```python
from build123d import *

# Parameters (mm, degrees)
SKETCH1_R           = 14.2875
BOSS_EXTRUDE1_DEPTH = 33.3375
SKETCH2_R           = 16.66875
BOSS_EXTRUDE2_DEPTH = 4.7625
FILLET1_R           = 3.175
SKETCH3_R           = 11.3109375
BOSS_EXTRUDE3_DEPTH = 4.7625
CUT_EXTRUDE1_START  = -4.7625
CUT_EXTRUDE1_DEPTH  = 4.7625


with BuildPart() as part:
    # Sketch1 → Boss-Extrude1 (new body)
    with BuildSketch(Plane.XY):
        Circle(SKETCH1_R)
    extrude(amount=BOSS_EXTRUDE1_DEPTH)

    # Sketch2 → Boss-Extrude2 (add)
    with BuildSketch(Plane(origin=(0, 0, 0), x_dir=(-1, 0, 0), z_dir=(0, 0, -1))):
        with Locations(Location((0, 0, 0), (0, 0, 180))):
            Circle(SKETCH2_R)
    extrude(amount=BOSS_EXTRUDE2_DEPTH)

    # Fillet1
    fillet1_edges = [part.edges().sort_by_distance(p)[0] for p in [
        (-16.66875, 0, -4.7625),
    ]]
    fillet(fillet1_edges, radius=FILLET1_R)

    # Sketch3 → Boss-Extrude3 (add)
    with BuildSketch(Plane(origin=(0, 0, -4.7625), x_dir=(-1, 0, 0), z_dir=(0, 0, -1))):
        with Locations(Location((0, 0, 0), (0, 0, 180))):
            Circle(SKETCH3_R)
    extrude(amount=BOSS_EXTRUDE3_DEPTH)

    # Sketch4 → Cut-Extrude1 (cut)
    with BuildSketch(Plane.XY.offset(33.3375).offset(CUT_EXTRUDE1_START)):
        with BuildLine():
            Line((-7.540625, 12.135552351), (-6.074392361, 9.775861616))
            ThreePointArc((-6.074392361, 9.775861616), (0, 11.509375), (6.074392361, 9.775861616))
            Line((6.074392361, 9.775861616), (7.540625, 12.135552351))
            ThreePointArc((7.540625, 12.135552351), (14.2875, 0), (7.540625, -12.135552351))
            Line((7.540625, -12.135552351), (6.074392361, -9.775861616))
            ThreePointArc((6.074392361, -9.775861616), (0, -11.509375), (-6.074392361, -9.775861616))
            Line((-6.074392361, -9.775861616), (-7.540625, -12.135552351))
            ThreePointArc((-7.540625, -12.135552351), (-14.2875, 0), (-7.540625, 12.135552351))
        make_face()
    extrude(amount=CUT_EXTRUDE1_DEPTH, mode=Mode.SUBTRACT)


solid = part.part
```
Can you work these out from the model? Positions are in its coordinate system, mm. A direction names the side the tool comes from. Round coordinates to 2 decimals unless told otherwise and drop trailing zeros. Loops run counter-clockwise (first coordinate to the right, second up) from the corner with the lowest first, then second, coordinate; pieces in that order, holes last. Notation, with made-up numbers: M 37.5,25 L 76.5,25 A5 cw 76.5,32 Z; hole C 17,58.5 d5. An arc over 180 degrees is marked long. Answer in a Markdown table with one row per item.
1. Please list where these lines run through material, in increasing order: line 1 (Z direction, x = 7.5, y = 1.5) (3 decimals); line 2 (Y direction, x = 0, z = 13.5). Write a range as from..to.
Established:
| item | result |
|---|---|
| line 1 | -9.525..28.575 |
| line 2 | -14.29..14.29 |
2. Thinking about a two-plate mould opening in X: for faces 6 (the face through (-6.818, 10.972, 30.923)), 7 (the face through (6.818, -10.972, 30.923)), 8 (the face through (-0.09, 11.51, 30.92)), which applies, pulls with the +X half, pulls with the -X half, needs draft (parallel to the pull), parting line crosses it, or undercut?
Established:
| item | result |
|---|---|
| face 6 | pulls with the -X half |
| face 7 | pulls with the +X half |
| face 8 | undercut |
3. On a 3-axis mill with a long thin cutter (end or side, diameter ignored), from which of +Z, -Z, +X, -X, +Y, -Y can I reach the whole of each face in a straight line? I mean faces 1 (the face through (-1.472, -11.215, -7.11)), 2 (the face through (0, 0, -9.525)), 3 (the face through (6.593, -12.675, 16.435)), 4 (the face through (6.8, 10.94, 30.92)), 5 (the face through (-6.8, -10.94, 30.92)). Say none if no direction works.
Established:
| item | result |
|---|---|
| face 1 | -Z |
| face 2 | -Z, +X, -X, +Y, -Y |
| face 3 | +Z |
| face 4 | +Z, +X |
| face 5 | +Z, -X |
4. If we section it at C-C, the plane z = 19.5: Please give me the cut outline in (x, y) (1 decimal).
Established:
| item | result |
|---|---|
| outline | C 0,0 d28.6 |
5. I'm going to push flat-ended pins straight in: pin 1 Ø1 at (y, z) = (-9, 25.5) entering from +X; pin 2 Ø1 at (x, y) = (-6.5, -7) entering from +Z (3 decimals); pin 3 Ø10 at (y, z) = (-1.5, 27) entering from -X. Where does each tip first touch, or does it pass through?
Established:
| item | result |
|---|---|
| pin 1 | x = 11.48 |
| pin 2 | z = 28.575 |
| pin 3 | x = -14.29 |
